Build history of the part. All positions in model axes, mm. Face numbers are marked on the shaded views. A direction names the side the tool comes from. Round coordinates to 2 decimals unless told otherwise and drop trailing zeros. Write each loop counter-clockwise with the first axis right and the second up, starting at its lowest first coordinate (ties: lowest second). Pieces come first, ordered by that corner, then holes. Notation, with made-up numbers: M -32.5,71.5 L -27.5,71.5 A18 ccw -27.5,75.5 Z; hole C 89.5,74.25 d8. An arc over 180 degrees is marked long. Use a Markdown table: item, result.
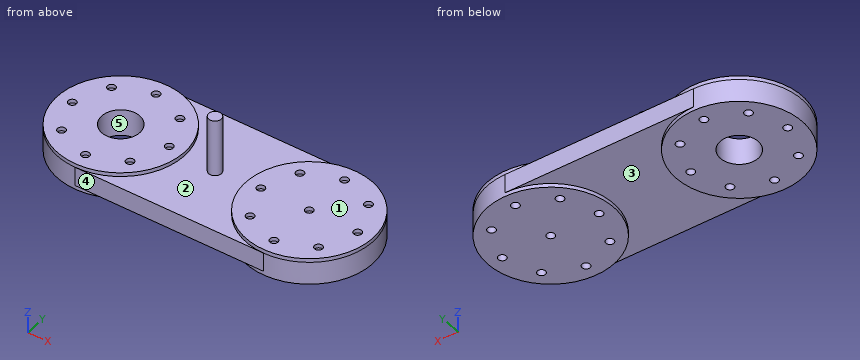
from build123d import *

# Parameters (mm, degrees)
SKETCH_1_W               = 150
SKETCH_1_H               = 100
SHORT_ARM_BODY_DEPTH     = 15
SKETCH_1_17_R            = 5
EXTRUDE_8_DEPTH          = 45
SKETCH_1_30_R            = 50
SKETCH_1_30_R_2          = 3.175
EXTRUDE_10_DEPTH         = 3
SKETCH_1_31_R            = 50
CUT_EXTRUDE_1_DEPTH      = 88
CUT_EXTRUDE_1_DEPTH_BACK = 59
SKETCH_1_33_R            = 50
SKETCH_1_33_R_2          = 3.175
EXTRUDE_12_DEPTH         = 3
EXTRUDE_12_DEPTH_BACK    = 18
SKETCH_3_R               = 15
CUT_EXTRUDE_3_DEPTH      = 98


with BuildPart() as part:
    # Sketch 1 → short_arm_body (new body)
    with BuildSketch(Plane.XY):
        with Locations((-75, 50)):
            Rectangle(SKETCH_1_W, SKETCH_1_H)
    extrude(amount=-SHORT_ARM_BODY_DEPTH)

    # Sketch 1_17 → Extrude 8 (add)
    with BuildSketch(Plane.XY):
        with Locations((-75, 50)):
            Circle(SKETCH_1_17_R)
    extrude(amount=EXTRUDE_8_DEPTH)

    # Sketch 1_30 → Extrude 10 (add)
    with BuildSketch(Plane.XY):
        with Locations((0, 50)):
            Circle(SKETCH_1_30_R)
        with Locations((0, 11.469660941)):
            Circle(SKETCH_1_30_R_2, mode=Mode.SUBTRACT)
        with BuildLine():
            Line((0, 25), (0, 46.825))
            ThreePointArc((0, 46.825), (-2.24506403, 47.75493597), (-3.175, 50))
            Line((-3.175, 50), (-25, 50))
            ThreePointArc((-25, 50), (17.67766953, 67.67766953), (0, 25))
        make_face(mode=Mode.SUBTRACT)
        with Locations((0, 88.530339059)):
            Circle(SKETCH_1_30_R_2, mode=Mode.SUBTRACT)
        with Locations((-38.530339059, 50)):
            Circle(SKETCH_1_30_R_2, mode=Mode.SUBTRACT)
        with Locations((-27.24506403, 77.24506403)):
            Circle(SKETCH_1_30_R_2, mode=Mode.SUBTRACT)
        with Locations((-27.24506403, 22.75493597)):
            Circle(SKETCH_1_30_R_2, mode=Mode.SUBTRACT)
        with Locations((27.24506403, 77.24506403)):
            Circle(SKETCH_1_30_R_2, mode=Mode.SUBTRACT)
        with Locations((38.530339059, 50)):
            Circle(SKETCH_1_30_R_2, mode=Mode.SUBTRACT)
        with Locations((27.24506403, 22.75493597)):
            Circle(SKETCH_1_30_R_2, mode=Mode.SUBTRACT)
    extrude(amount=EXTRUDE_10_DEPTH)

    # Sketch 1_31 → Cut-Extrude 1 (cut, two sides)
    with BuildSketch(Plane.XY) as cut_extrude_1_sk:
        with Locations((0, 50)):
            Circle(SKETCH_1_31_R)
        with Locations((-150, 50)):
            Circle(SKETCH_1_31_R)
    extrude(amount=CUT_EXTRUDE_1_DEPTH, mode=Mode.SUBTRACT)
    extrude(cut_extrude_1_sk.sketch, amount=-CUT_EXTRUDE_1_DEPTH_BACK, mode=Mode.SUBTRACT)

    # Sketch 1_33 → Extrude 12 (add, two sides)
    with BuildSketch(Plane.XY) as extrude_12_sk:
        with Locations((0, 50)):
            Circle(SKETCH_1_33_R)
        with Locations((38.530339059, 50)):
            Circle(SKETCH_1_33_R_2, mode=Mode.SUBTRACT)
        with Locations((27.24506403, 22.75493597)):
            Circle(SKETCH_1_33_R_2, mode=Mode.SUBTRACT)
        with Locations((0, 11.469660941)):
            Circle(SKETCH_1_33_R_2, mode=Mode.SUBTRACT)
        with Locations((-27.24506403, 22.75493597)):
            Circle(SKETCH_1_33_R_2, mode=Mode.SUBTRACT)
        with Locations((-38.530339059, 50)):
            Circle(SKETCH_1_33_R_2, mode=Mode.SUBTRACT)
        with Locations((-27.24506403, 77.24506403)):
            Circle(SKETCH_1_33_R_2, mode=Mode.SUBTRACT)
        with Locations((0, 88.530339059)):
            Circle(SKETCH_1_33_R_2, mode=Mode.SUBTRACT)
        with Locations((27.24506403, 77.24506403)):
            Circle(SKETCH_1_33_R_2, mode=Mode.SUBTRACT)
        with Locations((0, 50)):
            Circle(SKETCH_1_33_R_2, mode=Mode.SUBTRACT)
        with Locations((-150, 50)):
            Circle(SKETCH_1_33_R)
        with Locations((-111.469660941, 50)):
            Circle(SKETCH_1_33_R_2, mode=Mode.SUBTRACT)
        with Locations((-122.75493597, 22.75493597)):
            Circle(SKETCH_1_33_R_2, mode=Mode.SUBTRACT)
        with Locations((-150, 11.469660941)):
            Circle(SKETCH_1_33_R_2, mode=Mode.SUBTRACT)
        with Locations((-177.24506403, 22.75493597)):
            Circle(SKETCH_1_33_R_2, mode=Mode.SUBTRACT)
        with Locations((-188.530339059, 50)):
            Circle(SKETCH_1_33_R_2, mode=Mode.SUBTRACT)
        with Locations((-177.24506403, 77.24506403)):
            Circle(SKETCH_1_33_R_2, mode=Mode.SUBTRACT)
        with Locations((-150, 88.530339059)):
            Circle(SKETCH_1_33_R_2, mode=Mode.SUBTRACT)
        with Locations((-122.75493597, 77.24506403)):
            Circle(SKETCH_1_33_R_2, mode=Mode.SUBTRACT)
        with Locations((-150, 50)):
            Circle(SKETCH_1_33_R_2, mode=Mode.SUBTRACT)
    extrude(amount=EXTRUDE_12_DEPTH)
    extrude(extrude_12_sk.sketch, amount=-EXTRUDE_12_DEPTH_BACK)

    # Sketch 3 → Cut-Extrude 3 (cut)
    with BuildSketch(Plane(origin=(0, 0, -18), x_dir=(-1, 0, 0), z_dir=(0, 0, -1))):
        with Locations((150, 50)):
            Circle(SKETCH_3_R)
    extrude(amount=-CUT_EXTRUDE_3_DEPTH, mode=Mode.SUBTRACT)


solid = part.part
Q1. Cut at D-D on z = -11.5. Count the separate pieces of the cut face and the enclosed holes in it, and give its area (3 significant figures).
Response values:
| item | result |
|---|---|
| separate pieces | 1 |
| enclosed holes | 18 |
| area | 21,600 mm2 |
Q2. Cut at A-A on x = -75. Give the cut face in (y, z), and give its area (3 significant figures).
Response values:
| item | result |
|---|---|
| outline | M 0,-15 L 100,-15 L 100,0 L 55,0 L 55,45 L 45,45 L 45,0 L 0,0 Z |
| area | 1,950 mm2 |
Q3. Cut at B-B on y = 71.5. Give the cut face in (x, z), and give its area (3 significant figures).
Response values:
| item | result |
|---|---|
| outline | M -195.14,-18 L -104.86,-18 L -104.86,-15 L -45.14,-15 L -45.14,-18 L 45.14,-18 L 45.14,3 L -45.14,3 L -45.14,0 L -104.86,0 L -104.86,3 L -195.14,3 Z |
| area | 4,690 mm2 |
Q4. Drop flat-ended pins along their axis: P1, Ø8.5, axis at x = 0, y = 50, coming from the +Z side; P2, Ø5.5, axis at x = 27.25, y = 22.75, coming from the -Z side. Give the stop position or say it passes through.
Response values:
| item | result |
|---|---|
| P1 | stops at z = 3 |
| P2 | passes through |
Q5. Which spindle directions (+Z, -Z, +X, -X, +Y, -Y) get a long thin tool onto all of the face, cutting with end or side? Do the marked faces 1, 2 and 3. Say none if no direction does.
Response values:
| item | result |
|---|---|
| face 1 | +Z, +X, +Y, -Y |
| face 2 | +Z |
| face 3 | -Z |
Q6. Drill centre lines: L1, parallel to Y at x = -150, z = -5; L2, parallel to Y at x = 0, z = 1 (3 decimals); L3, parallel to Z at x = -146, y = 83. Where is each one in solid material? Low to high.
Response values:
| item | result |
|---|---|
| L1 | y = 0 to 8.29, 14.64 to 35, 65 to 85.36, 91.71 to 100 |
| L2 | y = 0 to 8.295, 14.645 to 46.825, 53.175 to 85.355, 91.705 to 100 |
| L3 | z = -18 to 3 |
Q7. Cut at C-C on x = -157.5. Give the cut face in (y, z).
Response values:
| item | result |
|---|---|
| outline | M 0.57,-18 L 37.01,-18 L 37.01,3 L 0.57,3 Z; M 62.99,-18 L 99.43,-18 L 99.43,3 L 62.99,3 Z |
Q8. Two-plate mould, pull along X, no slides. Class the marked faces 4 and 5: +X half, -X half, draft (parallel to the pull), parting line (faces both ways), or undercut.
Response values:
| item | result |
|---|---|
| face 4 | draft |
| face 5 | undercut |
